```python
from build123d import *

# Parameters (mm, degrees)
BOX_W          = 1
BOX_H          = 10
BOX_DEPTH      = 2
CYLINDER_R     = 2
CYLINDER_DEPTH = 10


with BuildPart() as cubo:
    # Box → Box (new body)
    with BuildSketch(Plane(origin=(-0.5, -5, 10), x_dir=(1, 0, 0), z_dir=(0, 0, 1))):
        with Locations((0.5, 5)):
            Rectangle(BOX_W, BOX_H)
    extrude(amount=BOX_DEPTH)


with BuildPart() as cut:
    # Cone → Cone (revolve)
    with BuildSketch(Plane(origin=(0, 0, 8), x_dir=(1, 0, 0), z_dir=(0, -1, 0))):
        Polygon((0, 0), (2, 0), (2.8, 4), (0, 4), align=None)
    revolve(axis=Axis((0, 0, 8), (0, 0, 1)))

    # Cut: cut Cubo
    add(cubo.part, mode=Mode.SUBTRACT)


with BuildPart() as fusion:
    # Cylinder → Cylinder (new body)
    with BuildSketch(Plane.XY):
        Circle(CYLINDER_R)
    extrude(amount=CYLINDER_DEPTH)

    # Fusion: union Cut
    add(cut.part)


solid = fusion.part
```
The model under review builds one solid part; all positions refer to its coordinate system, in mm. A direction names the side the tool comes from. Round coordinates to 2 decimals unless told otherwise and drop trailing zeros. Loops run counter-clockwise (first coordinate to the right, second up) from the corner with the lowest first, then second, coordinate; pieces in that order, holes last. Notation, with made-up numbers: M -1.5,66.5 L 12.5,66.5 A33 ccw 12.5,94.5 Z; hole C 8,-17.5 d7. An arc over 180 degrees is marked long. Answer as a JSON object with one key per item and string values.
(1) Take a section at C-C on z = 8.25. Give the boundary of the cut face in (x, y), and give its area (3 significant figures).
Resolved:
{"outline": "C 0,0 d4.1", "area": "13.2 mm²"}
(2) To check wall thickness, follow line 1 along Z through (x, y) = (-0.2, 0.5); line 2 along X through (y, z) = (1.7, 10.5); line 3 along X through (y, z) = (-0.65, 11.75). State the ranges of each line that lie inside material, in increasing order.
Resolved:
{"line 1": "0 to 10", "line 2": "-1.83 to -0.5, 0.5 to 1.83", "line 3": "-2.67 to -0.5, 0.5 to 2.67"}
(3) Clearance check with flat-ended pins moving along their axes: P1, Ø0.6, axis at y = -1, z = 11, coming from the +X side; P2, Ø1, axis at x = 0.5, z = 5.5, coming from the +Y side; P3, Ø0.5, axis at x = 0, y = 0, coming from the +Z side. State where each tip first meets the part, or that it passes through.
Resolved:
{"P1": "x = 2.52", "P2": "y = 2", "P3": "z = 10"}
(4) Take a section at B-B on x = 0. Give the boundary of the cut face in (y, z).
Resolved:
{"outline": "M -2.4,10 L -2,8 L -2,0 L 2,0 L 2,8 L 2.4,10 Z"}
(5) Tool access review of faces 5 (the flat face through (-0.5, 0, 11)), 6 (the flat face through (0, 0, 0)): name each direction out of +Z, -Z, +X, -X, +Y, -Y from which nothing blocks a thin tool from reaching the whole face with its end or side.
Resolved:
{"face 5": "+Z, +Y, -Y", "face 6": "-Z, +X, -X, +Y, -Y"}
(6) Take a section at D-D on z = 2.5. Give the boundary of the cut face in (x, y).
Resolved:
{"outline": "C 0,0 d4"}
(7) Draft analysis for pull direction X (two halves, no side actions). For faces 1 (the flat face through (0, 0, 10)), 2 (the cylindrical face through (0, -2, 4)), 3 (the flat face through (-1, 0, 12)), 4 (the flat face through (0.5, 0, 11)), state which applies: released by +X, released by -X, zero draft, split by the parting line, or undercut.
Resolved:
{"face 1": "undercut", "face 2": "split by the parting line", "face 3": "zero draft", "face 4": "undercut"}
(8) Take a section at A-A on y = 0. Give the boundary of the cut face in (x, z), and give its area (3 significant figures).
Resolved:
{"outline": "M -2.8,12 L -2,8 L -2,0 L 2,0 L 2,8 L 2.8,12 L 0.5,12 L 0.5,10 L -0.5,10 L -0.5,12 Z", "area": "49.2 mm²"}
